Solid Edge part; units mm, degrees
sketch "Sketch1" plane through (0, 0, 0) normal (0, -1, 0) x (1, 0, 0)
  circle A0 centre (0, 0) radius 3.5
extrude "Protrusion1" add sketch "Sketch1" against normal blind 5
sketch "Sketch2" plane through (0, 5, 0) normal (0, 1, 0) x (-1, 0, 0)
  circle A0 centre (0, 0) radius 2.5
extrude "ExtrudedProtrusion_2" add sketch "Sketch2" along normal blind 20
cosmetic_thread "Thread_1" thread depth 20
fillet "Round_1" radius 0.2 1 edges at (-3.5, 0, 0)
sketch "Sketch3" plane through (0, 0, 0) normal (0, -1, 0) x (1, 0, 0)
  line L0 (0, 1.4434) -> (-1.25, 0.7217)
  line L1 (-1.25, 0.7217) -> (-1.25, -0.7217)
  line L2 (-1.25, -0.7217) -> (0, -1.4434)
  line L3 (0, -1.4434) -> (1.25, -0.7217)
  line L4 (1.25, -0.7217) -> (1.25, 0.7217)
  line L5 (1.25, 0.7217) -> (0, 1.4434)
extrude "ExtrudedCutout_2" cut sketch "Sketch3" against normal blind 2.3
properties material "Steel"
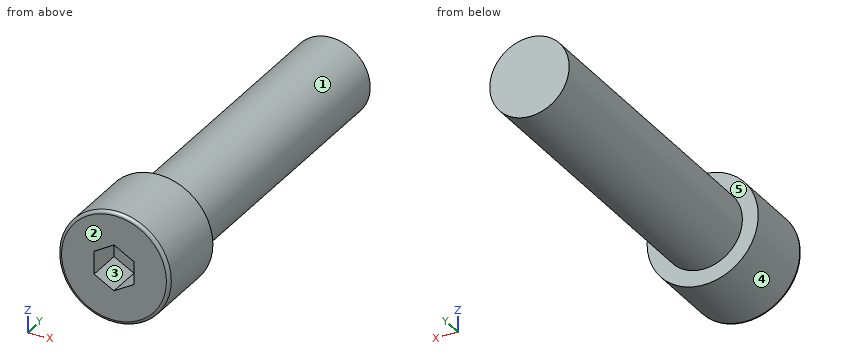
Part model, mm, in its own coordinate system. Face numbers are marked on the shaded views. A direction names the side the tool comes from. Coordinates: 2 decimals unless noted, no trailing zeros. Order: outer loops, then holes, each group sorted by start corner. A loop starts at its lowest first (then second) coordinate and runs counter-clockwise, first axis right, second up. Notation, with made-up numbers: (40, 23.5) - (96, 23.5) arc R28 ccw to (96, 51.5) - close; hole circle Ø3 at (-14.5, -40). An arc over 180 degrees is marked (long way). Return JSON: item names as keys, results as strings. Group by question number.
Item 1: Cut at B-B (y = 17.75). List the corners of the cut face in (x, z).
Item 2: Pull direction Z, two halves, no side cores. Call the marked faces 1, 2 and 3: pulls with the +Z half, pulls with the -Z half, needs draft (parallel to the pull), parting line crosses it, or undercut.
Item 3: Cut at C-C (y = 3). List the corners of the cut face in (x, z), plus the area to 3 significant figures.
Item 4: Pin check, flat tips, straight feed: pin 1 (1 mm diameter, centred on x = -1.5, z = 1.5, fed in from -Y); pin 2 (4 mm diameter, centred on y = 16.5, z = -1, fed in from +X); pin 3 (2 mm diameter, centred on x = -1.5, y = 5, fed in from -Z). Stop position of each tip, or through.
Item 5: Cut at A-A (z = 0). List the corners of the cut face in (x, y), plus the area to 3 significant figures.
Item 6: Drill centre lines: probe 1 along Z at (x, y) = (0, 20.25); probe 2 along Y at (x, z) = (2.25, 2); probe 3 along X at (y, z) = (17.5, 0.75). Where is each one in solid material? Low to high. Write a range as from..to.
Item 7: Which spindle directions (+Z, -Z, +X, -X, +Y, -Y) get a long thin tool onto all of the face, cutting with end or side? Do the marked faces 4 and 5. Say none if no direction does.
Check values:
{
 "1": {"outline": "circle Ø5 at (0, 0)"},
 "2": {"face 1": "parting line crosses it", "face 2": "needs draft", "face 3": "undercut"},
 "3": {"outline": "circle Ø7 at (0, 0)", "area": "38.5 mm2"},
 "4": {"pin 1": "stops at y = 0", "pin 2": "stops at x = 2.5", "pin 3": "stops at z = -3.46"},
 "5": {"outline": "(-3.5, 0.2) arc R0.2 ccw to (-3.3, 0) - (-1.25, 0) - (-1.25, 2.3) - (1.25, 2.3) - (1.25, 0) - (3.3, 0) arc R0.2 ccw to (3.5, 0.2) - (3.5, 5) - (2.5, 5) - (2.5, 25) - (-2.5, 25) - (-2.5, 5) - (-3.5, 5) - close", "area": "129 mm2"},
 "6": {"probe 1": "z = -2.5..2.5", "probe 2": "y = 0..5", "probe 3": "x = -2.38..2.38"},
 "7": {"face 4": "+Y, -Y", "face 5": "+Y"}
}
